Source: three-view drawing plus pictorial views. Frame: mm from the lowest corner of the part. A direction names the side the tool comes from. Round coordinates to 2 decimals unless told otherwise and drop trailing zeros. Loops run counter-clockwise (first coordinate to the right, second up) from the corner with the lowest first, then second, coordinate; pieces in that order, holes last. Notation, with made-up numbers: (18.5, -35.5) -> (55.5, -35.5) arc R24 ccw to (55.5, -22.5) -> close; hole circle Ø9 at (62, 17). An arc over 180 degrees is marked (long way). Answer in a Markdown table with one row per item.
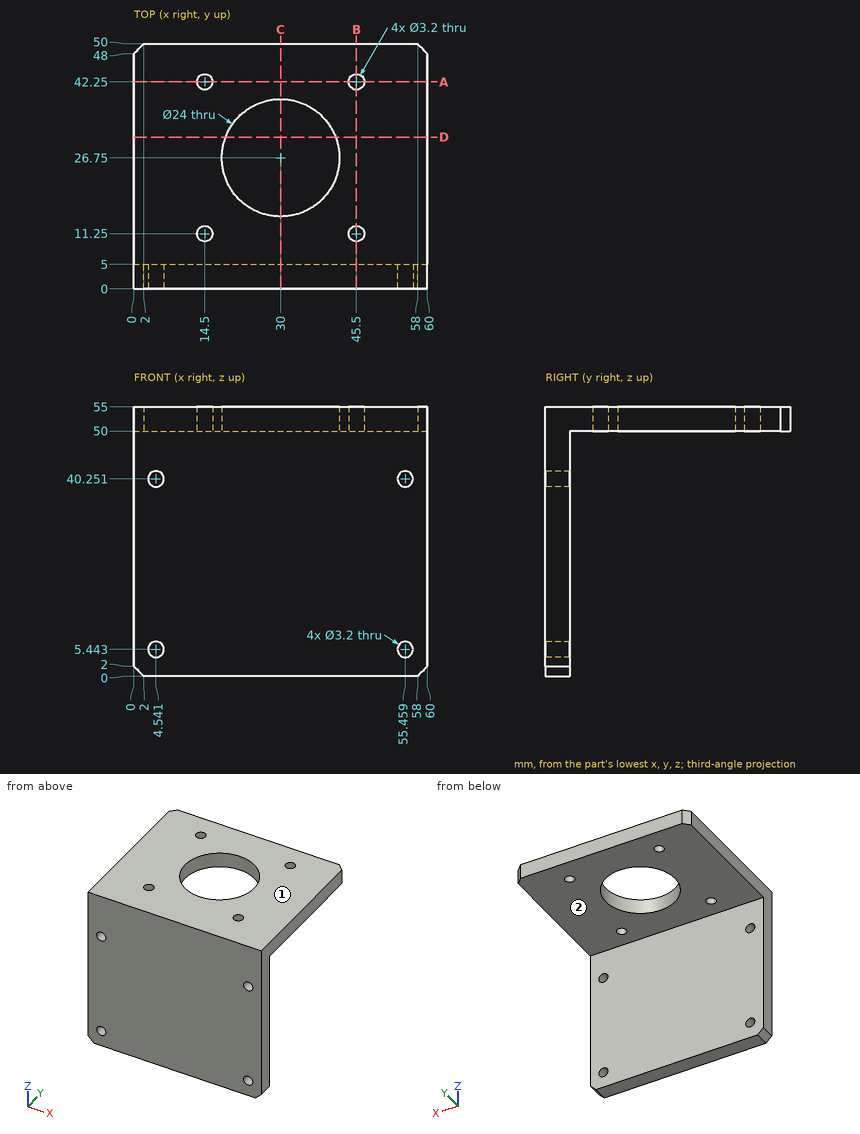
Item 1: Cut plane C-C (x = 30). Output: boundary loops of the cut face in (y, z), then the cut area to 3 significant figures.
Answer:
| item | result |
|---|---|
| outline | (0, 0) -> (5, 0) -> (5, 50) -> (14.75, 50) -> (14.75, 55) -> (0, 55) -> close; (38.75, 50) -> (50, 50) -> (50, 55) -> (38.75, 55) -> close |
| area | 380 mm² |
Item 2: Cut plane B-B (x = 45.5). Output: boundary loops of the cut face in (y, z), then the cut area to 3 significant figures.
Answer:
| item | result |
|---|---|
| outline | (0, 0) -> (5, 0) -> (5, 50) -> (9.65, 50) -> (9.65, 55) -> (0, 55) -> close; (12.85, 50) -> (40.65, 50) -> (40.65, 55) -> (12.85, 55) -> close; (43.85, 50) -> (50, 50) -> (50, 55) -> (43.85, 55) -> close |
| area | 468 mm² |
Item 3: Line query: probe 1 along X at (y, z) = (11, 52); probe 2 along Y at (x, z) = (13, 12.5); probe 3 along Z at (x, y) = (22.5, 44). Output: solid intervals per line, ascending. Write a range as [from, to].
Answer:
| item | result |
|---|---|
| probe 1 | x = [0, 12.92], [16.08, 43.92], [47.08, 60] |
| probe 2 | y = [0, 5] |
| probe 3 | z = [50, 55] |
Item 4: Cut plane A-A (y = 42.25). Output: boundary loops of the cut face in (x, z).
Answer:
| item | result |
|---|---|
| outline | (0, 50) -> (12.9, 50) -> (12.9, 55) -> (0, 55) -> close; (16.1, 50) -> (43.9, 50) -> (43.9, 55) -> (16.1, 55) -> close; (47.1, 50) -> (60, 50) -> (60, 55) -> (47.1, 55) -> close |
Item 5: Cut plane D-D (y = 31). Output: boundary loops of the cut face in (x, z).
Answer:
| item | result |
|---|---|
| outline | (0, 50) -> (18.78, 50) -> (18.78, 55) -> (0, 55) -> close; (41.22, 50) -> (60, 50) -> (60, 55) -> (41.22, 55) -> close |
Item 6: Pin query (flat end, axial travel): pin 1 Ø3.5 at (x, y) = (45.5, 11.25) entering from -Z; pin 2 Ø1.5 at (x, z) = (38, 46) entering from +Y. Return the tip coordinate at first contact, or that it passes through.
Answer:
| item | result |
|---|---|
| pin 1 | stops at z = 50 |
| pin 2 | stops at y = 5 |
Item 7: Reachability of the marked faces 1 and 2 from +Z, -Z, +X, -X, +Y, -Y: full face, straight path, thin tool, end or side. Return the list, or none.
Answer:
| item | result |
|---|---|
| face 1 | +Z, +X, -X, +Y, -Y |
| face 2 | -Z, +X, -X, +Y |
